The figure shows three views and two pictorial views of one solid part (mm, origin at its lowest corner). Answer the questions. A direction names the side the tool comes from. Coordinates: 2 decimals unless noted, no trailing zeros. Loops run counter-clockwise (first coordinate to the right, second up) from the corner with the lowest first, then second, coordinate; pieces in that order, holes last. Notation, with made-up numbers: (-18.75, 0) - (-11.75, 0) arc R19 cw to (-11.75, 4) - close; hole circle Ø8 at (89, -29.75). An arc over 180 degrees is marked (long way). Return JSON: item names as keys, results as strings. Group by question number.
1. Which of the six approach directions +Z, -Z, +X, -X, +Y, -Y give full straight-line access (tool end or side, diameter ignored) to the marked faces 4, 5 and 6?
2. The mould has two halves that part along Z. Classify the marked faces 1, 2 and 3: pulls with the +Z half, pulls with the -Z half, needs draft (parallel to the pull), parting line crosses it, or undercut.
3. Section D-D (y = 14.25) is taken. Write down the section's boundary in (x, z) (1 decimal).
4. Find the intervals of material crossed by line 1 along Y through (x, z) = (7.5, 55); line 2 along X through (y, z) = (26.25, 22); line 3 along Z through (x, y) = (15, 5.5), in increasing order.
5. Section B-B (x = 4.75) is taken. Write down the section's boundary in (y, z).
6. Section A-A (z = 39) is taken. Write down the section's boundary in (x, y).
7. Each of these flat-tipped pins is pushed along its axis until it touches: P1, Ø3.5, axis at x = 14.5, y = 10.5, coming from the -Z side; P2, Ø7, axis at y = 15.35, z = 15.15, coming from the +X side. Where does it stop, or does it pass through?
8. Section C-C (z = 46) is taken. Write down the section's boundary in (x, y), and give its area (3 significant figures).
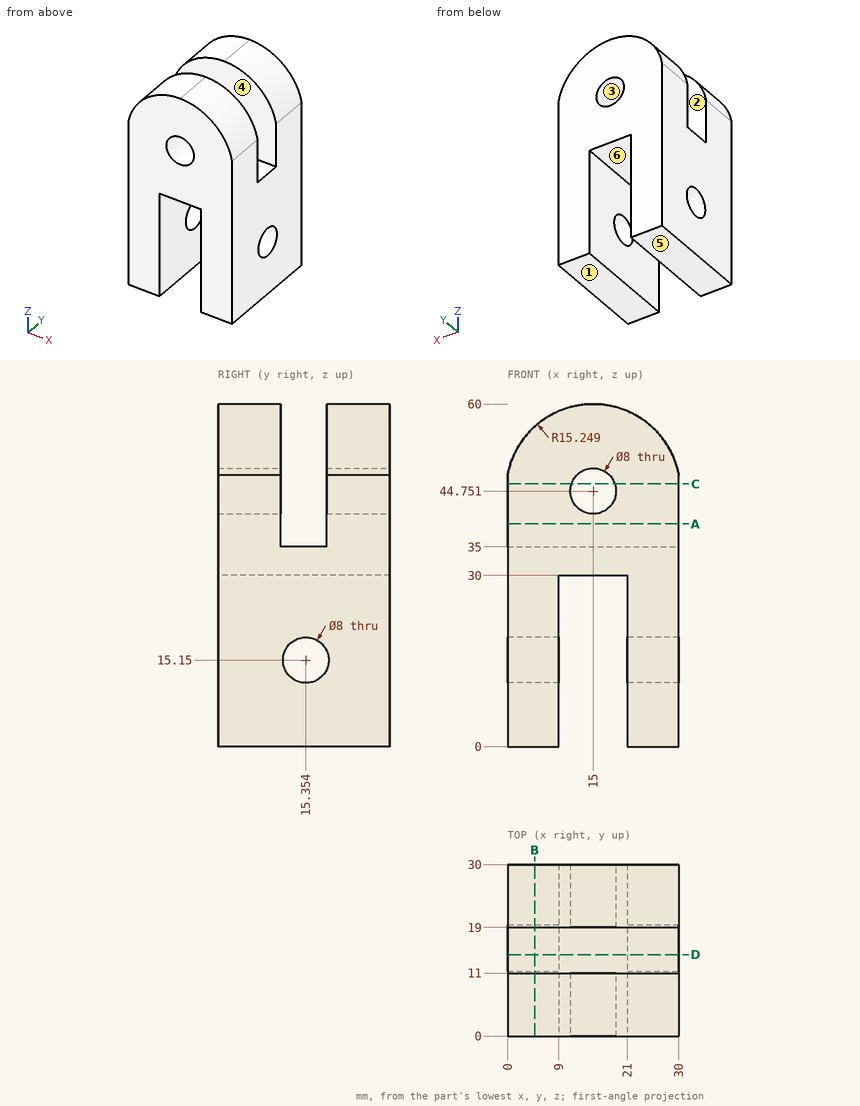
The answers:
{
 "1": {"face 4": "+Z, +X, -X", "face 5": "-Z, +X, -X, +Y, -Y", "face 6": "-Z, +Y, -Y"},
 "2": {"face 1": "pulls with the -Z half", "face 2": "needs draft", "face 3": "undercut"},
 "3": {"outline": "(0, 0) - (9, 0) - (9, 11.3) - (0, 11.3) - close; (0, 19) - (9, 19) - (9, 30) - (21, 30) - (21, 19) - (30, 19) - (30, 35) - (0, 35) - close; (21, 0) - (30, 0) - (30, 11.3) - (21, 11.3) - close"},
 "4": {"line 1": "y = 0 to 11, 19 to 30", "line 2": "x = 0 to 9, 21 to 30", "line 3": "z = 30 to 40.75, 48.75 to 60"},
 "5": {"outline": "(0, 0) - (30, 0) - (30, 56.04) - (19, 56.04) - (19, 35) - (11, 35) - (11, 56.04) - (0, 56.04) - close; hole circle Ø8 at (15.35, 15.15)"},
 "6": {"outline": "(0, 0) - (30, 0) - (30, 11) - (0, 11) - close; (0, 19) - (30, 19) - (30, 30) - (0, 30) - close"},
 "7": {"P1": "stops at z = 30", "P2": "passes through"},
 "8": {"outline": "(0, 0) - (11.2, 0) - (11.2, 11) - (0, 11) - close; (0, 19) - (11.2, 19) - (11.2, 30) - (0, 30) - close; (18.8, 0) - (30, 0) - (30, 11) - (18.8, 11) - close; (18.8, 19) - (30, 19) - (30, 30) - (18.8, 30) - close", "area": "493 mm2"}
}
